```python
from build123d import *

# Parameters (mm, degrees)
BOSS_EXTRUDE1_DEPTH = 35
SKETCH3_W           = 97
SKETCH3_H           = 201
BOSS_EXTRUDE2_DEPTH = 5
FILLET1_R           = 10
SKETCH4_R           = 2.75
CUT_EXTRUDE1_DEPTH  = 10
CHAMFER3_SIZE       = 2.7
CHAMFER3_SIZE2      = 3.8
CHAMFER4_SIZE       = 2.7
CHAMFER4_SIZE2      = 3.8


with BuildPart() as part:
    # Sketch1 → Boss-Extrude1 (new body)
    with BuildSketch(Plane(origin=(0, 0, 0), x_dir=(1, 0, 0), z_dir=(0, 1, 0))):
        Polygon((-45.5, -97.5), (-45.5, -100.5), (-48.5, -100.5), (-48.5, 100.5), (48.5, 100.5), (48.5, -100.5), (45.5, -100.5), (45.5, -97.5), (45.5, 97.5), (-45.5, 97.5), align=None)
    extrude(amount=BOSS_EXTRUDE1_DEPTH)

    # Sketch3 → Boss-Extrude2 (add)
    with BuildSketch(Plane.XZ):
        Rectangle(SKETCH3_W, SKETCH3_H)
    extrude(amount=BOSS_EXTRUDE2_DEPTH)

    # Fillet1
    fillet1_edges = [part.edges().sort_by_distance(p)[0] for p in [
        (47, 35, 100.5),
        (-47, 35, 100.5),
    ]]
    fillet(fillet1_edges, radius=FILLET1_R)

    # Sketch4 → Cut-Extrude1 (cut)
    with BuildSketch(Plane(origin=(0, 0, 0), x_dir=(1, 0, 0), z_dir=(0, 1, 0))):
        with Locations(Location((-3.5, 60, 0), (0, 0, 270))):
            Circle(SKETCH4_R)
        with Locations(Location((-3.5, -60, 0), (0, 0, 270))):
            Circle(SKETCH4_R)
    extrude(amount=-CUT_EXTRUDE1_DEPTH, mode=Mode.SUBTRACT)

    # Chamfer3
    chamfer3_edges = [part.edges().sort_by_distance(p)[0] for p in [
        (-3.5, 0, 57.25),
    ]]
    chamfer3_side = [part.faces().sort_by_distance(p)[0] for p in [
        (0.009254512, 0, 1.50396622),
    ]]
    chamfer(chamfer3_edges, length=CHAMFER3_SIZE, length2=CHAMFER3_SIZE2, reference=chamfer3_side[0])

    # Chamfer4
    chamfer4_edges = [part.edges().sort_by_distance(p)[0] for p in [
        (-3.5, 0, -62.75),
    ]]
    chamfer4_side = [part.faces().sort_by_distance(p)[0] for p in [
        (0.022889878, 0, 1.276677255),
    ]]
    chamfer(chamfer4_edges, length=CHAMFER4_SIZE, length2=CHAMFER4_SIZE2, reference=chamfer4_side[0])


solid = part.part
```
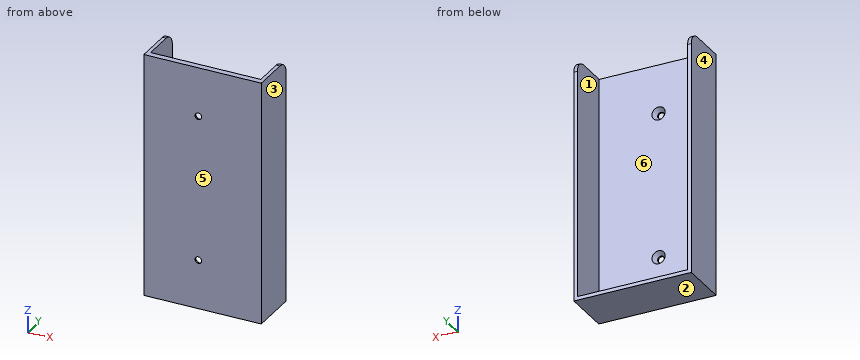
Part model, mm, in its own coordinate system. Face numbers are marked on the shaded views. A direction names the side the tool comes from. Give positions to 0.01 mm unless a question says otherwise; leave off trailing zeros. Order: outer loops, then holes, each group sorted by start corner. A loop starts at its lowest first (then second) coordinate and runs counter-clockwise, first axis right, second up. Notation, with made-up numbers: (10, -39.5) - (67, -39.5) arc R28 cw to (67, -2.5) - close; hole circle Ø11 at (-18, 15). An arc over 180 degrees is marked (long way). Use one line per item in the form item = value.
Item 1: Probe probe 1 along Z at (x, y) = (-3, -4); probe 2 along X at (y, z) = (16, 38.5); probe 3 along Z at (x, y) = (-15, 0.5). List the from-to ranges inside material, lowest first. Write a range as from..to.
Solution:
probe_1 = -100.5..-62.7, -57.3..57.3, 62.7..100.5
probe_2 = -48.5..-45.5, 45.5..48.5
probe_3 = -100.5..-97.5
Item 2: Two-plate mould, pull along X, no slides. Class the marked faces 1, 2, 3 and 4: released by +X, released by -X, zero draft, split by the parting line, or undercut.
Solution:
face_1 = undercut
face_2 = zero draft
face_3 = released by +X
face_4 = released by -X
Item 3: Slice it at B-B on z = 60. Give the cut face in (x, y).
Solution:
outline = (-48.5, -5) - (-6.25, -5) - (-6.25, -3.8) - (-8.95, 0) - (-45.5, 0) - (-45.5, 35) - (-48.5, 35) - close; (-0.75, -5) - (48.5, -5) - (48.5, 35) - (45.5, 35) - (45.5, 0) - (1.95, 0) - (-0.75, -3.8) - close
Item 4: Slice it at C-C on y = 23. Give the cut face in (x, z), and give its area (3 significant figures).
Solution:
outline = (-48.5, -100.5) - (48.5, -100.5) - (48.5, 100.5) - (45.5, 100.5) - (45.5, -97.5) - (-45.5, -97.5) - (-45.5, 100.5) - (-48.5, 100.5) - close
area = 1,480 mm2
Item 5: Which spindle directions (+Z, -Z, +X, -X, +Y, -Y) get a long thin tool onto all of the face, cutting with end or side? Do the marked faces 5 and 6. Say none if no direction does.
Solution:
face_5 = +Z, -Z, +X, -X, -Y
face_6 = +Z, +Y
Item 6: Slice it at D-D on z = -71.5. Give the cut face in (x, y), and give its area (3 significant figures).
Solution:
outline = (-48.5, -5) - (48.5, -5) - (48.5, 35) - (45.5, 35) - (45.5, 0) - (-45.5, 0) - (-45.5, 35) - (-48.5, 35) - close
area = 695 mm2
Item 7: Slice it at A-A on x = -3.5. Give the cut face in (y, z), and give its area (3 significant figures).
Solution:
outline = (-5, -100.5) - (35, -100.5) - (35, -97.5) - (0, -97.5) - (0, -65.45) - (-3.8, -62.75) - (-5, -62.75) - close; (-5, -57.25) - (-3.8, -57.25) - (0, -54.55) - (0, 54.55) - (-3.8, 57.25) - (-5, 57.25) - close; (-5, 62.75) - (-3.8, 62.75) - (0, 65.45) - (0, 100.5) - (-5, 100.5) - close
area = 1,030 mm2
Item 8: Pin check, flat tips, straight feed: pin 1 Ø4.5 at (x, z) = (-3.5, -60) entering from -Y; pin 2 Ø6.5 at (x, z) = (-3.5, 60) entering from +Y; pin 3 Ø8 at (x, y) = (-38, 19) entering from +Z; pin 4 Ø1.5 at (x, z) = (-24, 31) entering from +Y. Stop position of each tip, or through.
Solution:
pin_1 = through
pin_2 = -3.1
pin_3 = -97.5
pin_4 = 0
